Can you work these out from the model? Positions are in its coordinate system, mm. Face numbers are marked on the shaded views. A direction names the side the tool comes from. Round coordinates to 2 decimals unless told otherwise and drop trailing zeros. Loops run counter-clockwise (first coordinate to the right, second up) from the corner with the lowest first, then second, coordinate; pieces in that order, holes last.
from build123d import *

# Parameters (mm, degrees)
SKETCH1_R           = 10
BOSS_EXTRUDE1_DEPTH = 25
SKETCH4_R           = 1.5
BOSS_EXTRUDE2_DEPTH = 20
SKETCH6_W           = 7.254775406
SKETCH6_H           = 3
BOSS_EXTRUDE3_DEPTH = 25
CUT_EXTRUDE1_DEPTH  = 31.822070015
SKETCH7_R           = 1.75
CUT_EXTRUDE2_DEPTH  = 30.983328701


# Read off the part's stored shape, not the designer's step: Boundary-Cut1
with BuildPart() as part:
    # Sketch1 → Boss-Extrude1 (new body)
    with BuildSketch(Plane(origin=(0, 0, 0), x_dir=(1, 0, 0), z_dir=(0, 1, 0))):
        with Locations(Location((0, 0, 0), (0, 0, 270))):
            Circle(SKETCH1_R)
    extrude(amount=BOSS_EXTRUDE1_DEPTH)

    # Boundary-Cut1 outline → Boundary-Cut1 (revolve, cut)
    with BuildSketch(Plane.XY):
        Polygon((0, 5), (5, 5), (6.5, 25), (0, 25), align=None)
    revolve(axis=Axis((0, 0, 0), (0, 1, 0)), mode=Mode.SUBTRACT)

    # Sketch4 → Boss-Extrude2 (add)
    with BuildSketch(Plane(origin=(0, 5, 0), x_dir=(1, 0, 0), z_dir=(0, 1, 0))):
        with Locations(Location((0, 0, 0), (0, 0, 90))):
            Circle(SKETCH4_R)
    extrude(amount=BOSS_EXTRUDE2_DEPTH)

    # Sketch6 → Boss-Extrude3 (add)
    with BuildSketch(Plane(origin=(0, 0, 0), x_dir=(1, 0, 0), z_dir=(0, 1, 0))):
        with Locations((-11.372612297, 1.5)):
            Rectangle(SKETCH6_W, SKETCH6_H)
    boss_extrude3 = extrude(amount=BOSS_EXTRUDE3_DEPTH)

    # Sketch5 → Cut-Extrude1 (cut, through all)
    with BuildSketch(Plane(origin=(0, 25, 0), x_dir=(1, 0, 0), z_dir=(0, 1, 0))):
        with BuildLine():
            Line((-1.5, 0), (-10, 0))
            ThreePointArc((-10, 0), (0, -10), (10, 0))
            Line((10, 0), (1.5, 0))
            ThreePointArc((1.5, 0), (0, -1.5), (-1.5, 0))
        make_face()
    extrude(amount=-CUT_EXTRUDE1_DEPTH, mode=Mode.SUBTRACT)

    # Sketch7 → Cut-Extrude2 (cut, through all)
    with BuildSketch(Plane(origin=(0, 0, -3), x_dir=(-1, 0, 0), z_dir=(0, 0, -1))):
        with Locations((12.269696007, 5)):
            Circle(SKETCH7_R)
        with Locations((12.269696007, 20)):
            Circle(SKETCH7_R)
    cut_extrude2 = extrude(amount=-CUT_EXTRUDE2_DEPTH, mode=Mode.SUBTRACT)

    # Mirror1: Boss-Extrude3, Cut-Extrude2 across plane
    add(boss_extrude3.mirror(Plane(origin=(0, 0, 0), x_dir=(0, 0, 1), z_dir=(1, 0, 0))))
    add(cut_extrude2.mirror(Plane(origin=(0, 0, 0), x_dir=(0, 0, 1), z_dir=(1, 0, 0))), mode=Mode.SUBTRACT)


solid = part.part
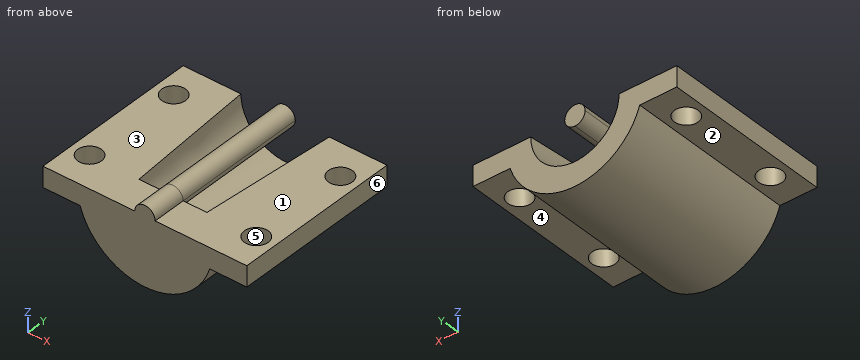
(1) If we section it at D-D, the plane z = -0.5: State how many separate pieces and enclosed holes the cut face has, then the cut area to 3 significant figures.
Worked answers:
separate pieces: 1
enclosed holes: 4
area: 539 mm2
(2) If I drill on line 1 (X direction, y = 4, z = -0.5); line 2 (X direction, y = 3.5, z = -2.75); line 3 (Z direction, x = -12.5, y = 8), over which ranges is the centre line in solid material (lowest first)?
Worked answers:
line 1: x = -15 to -13.71, -10.83 to 10.83, 13.71 to 15
line 2: x = -15 to -13.17, -11.37 to 11.37, 13.17 to 15
line 3: z = -3 to 0
(3) Will these pins go through, and if not, where does the flat tip stop? P1, Ø3, axis at x = 12.27, y = 5, coming from the -Z side; P2, Ø4.5, axis at x = -13, y = 16, coming from the -Z side; P3, Ø5, axis at x = 4.5, y = 14, coming from the -Z side; P4, Ø4, axis at x = -10.5, y = 10.5, coming from the +Z side.
Worked answers:
P1: passes through
P2: stops at z = -3
P3: stops at z = -9.8
P4: stops at z = 0
(4) If we section it at C-C, the plane x = 11.25: List the corners of the cut face in (y, z) for me, then the cut area to 3 significant figures.
Worked answers:
outline: (0, -3) - (3.58, -3) - (3.58, 0) - (0, 0) - close; (6.42, -3) - (18.58, -3) - (18.58, 0) - (6.42, 0) - close; (21.42, -3) - (25, -3) - (25, 0) - (21.42, 0) - close
area: 57.9 mm2
(5) For the marked faces 1, 2 and 3, which set-ups out of +Z, -Z, +X, -X, +Y, -Y let a thin tool reach every point of the face, with its end or its side?
Worked answers:
face 1: +Z, +X, +Y, -Y
face 2: -Z, -X, +Y, -Y
face 3: +Z, -X, +Y, -Y
(6) If we section it at A-A, the plane y = 11.75: List the corners of the cut face in (x, z) for me.
Worked answers:
outline: (-15, -3) - (-9.54, -3) arc R10 ccw to (9.54, -3) - (15, -3) - (15, 0) - (5.51, 0) arc R5.51 cw to (-5.51, 0) - (-15, 0) - close; circle Ø3 at (0, 0)
(7) If we mould it in two halves opening along X, with no side actions, what happens to the marked faces 4, 5 and 6? For each: released by +X, released by -X, zero draft, split by the parting line, or undercut.
Worked answers:
face 4: zero draft
face 5: undercut
face 6: released by +X
(8) If we section it at B-B, the plane y = 20: List the corners of the cut face in (x, z) for me (3 decimals), then the cut area to 3 significant figures.
Worked answers:
outline: (-15, -3) - (-14.02, -3) - (-14.02, 0) - (-15, 0) - close; (-10.52, -3) - (-9.539, -3) arc R10 ccw to (9.539, -3) - (10.52, -3) - (10.52, 0) - (6.125, 0) arc R6.125 cw to (-6.125, 0) - (-10.52, 0) - close; circle Ø3 at (0, 0); (14.02, -3) - (15, -3) - (15, 0) - (14.02, 0) - close
area: 115 mm2
